Autodesk Inventor part; units mm, degrees
ref_plane "YZ Plane" through (0, 0, 0) normal (1, 0, 0) x (0, 1, 0)
ref_plane "XZ Plane" through (0, 0, 0) normal (0, 1, 0) x (-1, 0, 0)
ref_plane "XY Plane" through (0, 0, 0) normal (0, 0, 1) x (1, 0, 0)
sketch "Sketch1" plane through (0, 0, 0) normal (0, 1, 0) x (-1, 0, 0)
  line L0 (0, 0) -> (-19.05, 0)
  line L1 (-19.05, 0) -> (-19.05, -45.72)
  line L2 (-19.05, -45.72) -> (0, -45.72)
  line L3 (0, -45.72) -> (0, 0)
  line L4 (-19.05, -15.24) -> (-22.225, -15.24)
  line L5 (-22.225, -15.24) -> (-22.225, -30.48)
  line L6 (-22.225, -30.48) -> (-19.05, -30.48)
  line L7 (-19.05, -30.48) -> (-19.05, -15.24)
  line L8 (0, -30.48) -> (3.175, -30.48)
  line L9 (3.175, -30.48) -> (3.175, -15.24)
  line L10 (3.175, -15.24) -> (0, -15.24)
  line L11 (0, -15.24) -> (0, -30.48)
  dimension "d0" = 19.05
  dimension "d1" = 45.72
  dimension "d2" = 3.175
  dimension "d3" = 15.24
  dimension "d4" = 3.175
  dimension "d5" = 15.24
  dimension "d6" = 15.24
extrude "Extrusion1" add sketch "Sketch1" along normal blind 3.175
sketch "Sketch2" plane through (0, 3.175, 0) normal (0, 1, 0) x (1, 0, 0)
  line L0 (-3.175, 30.48) -> (-3.175, 15.24)
  line L1 (19.05, 45.72) -> (0, 45.72)
  line L2 (5.2917, 45.72) -> (13.7583, 45.72)
  line L3 (13.7583, 45.72) -> (13.7583, 42.545)
  line L4 (13.7583, 42.545) -> (5.2917, 42.545)
  line L5 (5.2917, 42.545) -> (5.2917, 45.72)
  dimension "d9" = 8.4667
  dimension "d10" = 3.175
  dimension "d11" = 8.4667
extrude "Extrusion2" cut sketch "Sketch2" against normal blind 3.175
sketch "Sketch3" plane through (0, 3.175, 0) normal (0, 1, 0) x (1, 0, 0)
  line L0 (-3.175, 30.48) -> (-3.175, 15.24)
  line L1 (19.05, 45.72) -> (13.7583, 45.72)
  line L2 (3.525, 36.83) -> (15.525, 36.83)
  line L3 (15.525, 36.83) -> (15.525, 6.83)
  line L4 (15.525, 6.83) -> (3.525, 6.83)
  line L5 (3.525, 6.83) -> (3.525, 36.83)
  circle A0 centre (9.525, 4.33) radius 1.0541
  circle A1 centre (9.525, 39.33) radius 1.0541
  dimension "d14" = 12
  dimension "d15" = 30
  dimension "d16" = 6.7
  dimension "d17" = 8.89
  dimension "d18" = 2.1082
  dimension "d19" = 2.5
  dimension "d20" = 2.1082
  dimension "d21" = 2.5
  dimension "d22" = 6
  dimension "d23" = 6
extrude "Extrusion3" cut sketch "Sketch3" against normal blind 3.175
equation "\"d0\" = angleDepth - 2 * thick"
equation "\"d1\" = angleLength"
equation "\"d2\" = thick"
equation "\"d3\" = 0.333333 * angleLength"
equation "\"d4\" = thick"
equation "\"d5\" = 0.333333 * angleLength"
equation "\"d6\" = 0.333333 * angleLength"
equation "\"d7\" = thick"
equation "\"d9\" = 0.333333 * angleDepth"
equation "\"d10\" = thick"
equation "\"d11\" = 0.333333 * angleDepth"
equation "\"d12\" = thick"
equation "\"d14\" = servoWidth"
equation "\"d15\" = servoLength"
equation "\"d16\" = -0.5 * servoWidth + 0.5 * angleDepth"
equation "\"d17\" = servoOff"
equation "\"d18\" = servoHole"
equation "\"d19\" = -0.5 * servoLength + 0.5 * servoDist"
equation "\"d20\" = servoHole"
equation "\"d21\" = -0.5 * servoLength + 0.5 * servoDist"
equation "\"d22\" = 0.5 * servoWidth"
equation "\"d23\" = 0.5 * servoWidth"
equation "\"d24\" = thick"
equation "\"angleDepth\" = 25.4"
equation "\"thick\" = 3.175"
equation "\"angleLength\" = 45.72"
equation "\"servoLength\" = 30"
equation "\"servoWidth\" = 12"
equation "\"servoDist\" = 35"
equation "\"servoOff\" = 8.89"
equation "\"servoHole\" = 2.1082"
properties part number "AngleTop"
Verification items for the finished model (mm, model axes). A direction names the side the tool comes from. Round coordinates to 2 decimals unless told otherwise and drop trailing zeros. Write each loop counter-clockwise with the first axis right and the second up, starting at its lowest first coordinate (ties: lowest second). Pieces come first, ordered by that corner, then holes. Notation, with made-up numbers: (21.5, -12.5) -> (74.5, -12.5) arc R20 ccw to (74.5, 11.5) -> close; hole circle Ø3 at (58, 39.25). An arc over 180 degrees is marked (long way). Write each question's results on one line, items separated by ' | '.
Q1. Draft check along Z on faces 1 (the face through (3.525, 2, -22)), 2 (the face through (10.09, 1.61, -40.22)), 3 (the face through (18, 0, -23)), 4 (the face through (9, 2, 0)). Enter one of: released by +Z, released by -Z, zero draft, split by the parting line, or undercut.
Derived:
face 1: undercut | face 2: undercut | face 3: zero draft | face 4: released by +Z
Q2. Sectioned sample at C-C, the plane z = -14. Record the boundary of the cut face in (x, y) (3 decimals).
Derived:
outline: (0, 0) -> (3.525, 0) -> (3.525, 3.175) -> (0, 3.175) -> close; (15.525, 0) -> (19.05, 0) -> (19.05, 3.175) -> (15.525, 3.175) -> close
Q3. Sectioned sample at A-A, the plane z = -4.33. Record the boundary of the cut face in (x, y) (3 decimals).
Derived:
outline: (0, 0) -> (8.471, 0) -> (8.471, 3.175) -> (0, 3.175) -> close; (10.579, 0) -> (19.05, 0) -> (19.05, 3.175) -> (10.579, 3.175) -> close
Q4. Sectioned sample at D-D, the plane x = -0.5. Record the boundary of the cut face in (y, z) (3 decimals), and give its area (3 significant figures).
Derived:
outline: (0, -30.48) -> (3.175, -30.48) -> (3.175, -15.24) -> (0, -15.24) -> close | area: 48.4 mm²
Q5. Go/stop test with flat-tipped pins: pin 1 Ø1 at (y, z) = (1.5, -43.5) entering from +X; pin 2 Ø1 at (x, y) = (-2, 1) entering from +Z; pin 3 Ø1.6 at (x, y) = (11.5, 2) entering from -Z (3 decimals). Record where each tip stops, or that it passes through.
Derived:
pin 1: stops at x = 19.05 | pin 2: stops at z = -15.24 | pin 3: stops at z = -42.545
Q6. Thickness scan on probe 1 along X at (y, z) = (2.9, -11) (3 decimals); probe 2 along Z at (x, y) = (14.75, 2.1); probe 3 along Z at (x, y) = (11, 1.55) (3 decimals). Record the ranges inside material, lowest first.
Derived:
probe 1: x = 0 to 3.525, 15.525 to 19.05 | probe 2: z = -45.72 to -36.83, -6.83 to 0 | probe 3: z = -42.545 to -36.83, -6.83 to 0
Q7. Access from +Z, -Z, +X, -X, +Y, -Y to the whole of each face (thin tool, end or side, straight path). Record for faces 5 (the face through (21, 2, -15.24)), 6 (the face through (10, 2, -42.545)), 7 (the face through (21, 2, -30.48)), 8 (the face through (-2, 2, -30.48)), 9 (the face through (-2, 2, -15.24)).
Derived:
face 5: +Z, +X, +Y, -Y | face 6: -Z, +Y, -Y | face 7: -Z, +X, +Y, -Y | face 8: -Z, -X, +Y, -Y | face 9: +Z, -X, +Y, -Y
Q8. Sectioned sample at B-B, the plane y = 2.5. Record the boundary of the cut face in (x, z) (3 decimals).
Derived:
outline: (-3.175, -30.48) -> (0, -30.48) -> (0, -45.72) -> (5.292, -45.72) -> (5.292, -42.545) -> (13.758, -42.545) -> (13.758, -45.72) -> (19.05, -45.72) -> (19.05, -30.48) -> (22.225, -30.48) -> (22.225, -15.24) -> (19.05, -15.24) -> (19.05, 0) -> (0, 0) -> (0, -15.24) -> (-3.175, -15.24) -> close; hole (3.525, -36.83) -> (15.525, -36.83) -> (15.525, -6.83) -> (3.525, -6.83) -> close; hole circle Ø2.108 at (9.525, -39.33); hole circle Ø2.108 at (9.525, -4.33)
